Check sheet for the drawn part. Datum: minimum x, y, z corner. Units: mm. Give positions to 0.01 mm unless a question says otherwise; leave off trailing zeros. Write each loop counter-clockwise with the first axis right and the second up, starting at its lowest first coordinate (ties: lowest second). Pieces come first, ordered by that corner, then holes. Notation, with made-up numbers: (-3, -7) -> (44, -7) arc R14 cw to (44, 9) -> close; hole circle Ø6 at (-16.5, 30.5). An arc over 180 degrees is marked (long way). Use CSV: the item, a comma, the result in double quotes. Start each with the question number.
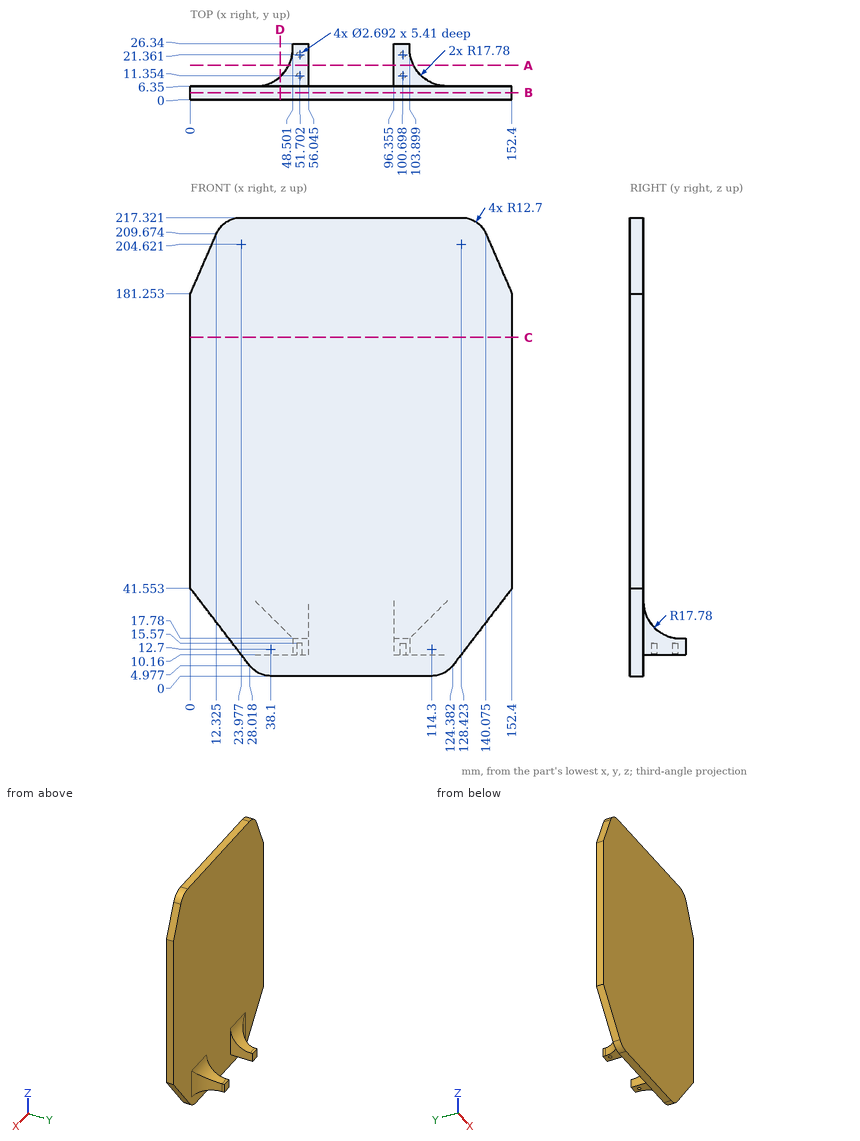
(1) Go/stop test with flat-tipped pins: pin 1 (6 mm diameter, centred on x = 104.5, y = 12, fed in from -Z); pin 2 (8 mm diameter, centred on x = 63.5, z = 62.5, fed in from +Y); pin 3 (2.5 mm diameter, centred on y = 25.5, z = 14.5, fed in from -X). Record where each tip stops, or that it passes through.
(2) Thickness scan on line 1 (Y direction, x = 143, z = 34.5); line 2 (X direction, y = 1.5, z = 30). Record the ranges inside material, lowest first. Write a range as from..to.
(3) Section check C-C on z = 160.5. Record the cut outline in (x, y).
(4) Section check A-A on y = 16.25. Record the cut outline in (x, z) (1 decimal).
(5) Section check B-B on y = 3.25. Record the cut outline in (x, z) (1 decimal), then the cut area to 3 significant figures.
(6) Section check D-D on x = 42.5. Record the cut outline in (y, z).
Data:
1,pin 1,"stops at z = 10.16"
1,pin 2,"stops at y = 6.35"
1,pin 3,"stops at x = 48.5"
2,line 1,"y = 0..6.35"
2,line 2,"x = 8.85..143.55"
3,outline,"(0, 0) -> (152.4, 0) -> (152.4, 6.35) -> (0, 6.35) -> close"
4,outline,"(46.7, 10.2) -> (56, 10.2) -> (56, 19.6) -> (46.7, 19.6) -> close; (96.4, 10.2) -> (105.7, 10.2) -> (105.7, 19.6) -> (96.4, 19.6) -> close"
5,outline,"(0, 41.6) -> (28, 5) arc R12.7 ccw to (38.1, 0) -> (114.3, 0) arc R12.7 ccw to (124.4, 5) -> (152.4, 41.6) -> (152.4, 181.3) -> (140.1, 209.7) arc R12.7 ccw to (128.4, 217.3) -> (24, 217.3) arc R12.7 ccw to (12.3, 209.7) -> (0, 181.3) -> close"
5,area,"31,200 mm2"
6,outline,"(0, 0) -> (6.35, 0) -> (6.35, 10.16) -> (10.81, 10.16) -> (10.81, 23.78) arc R17.78 cw to (6.35, 35.56) -> (6.35, 217.32) -> (0, 217.32) -> close"
